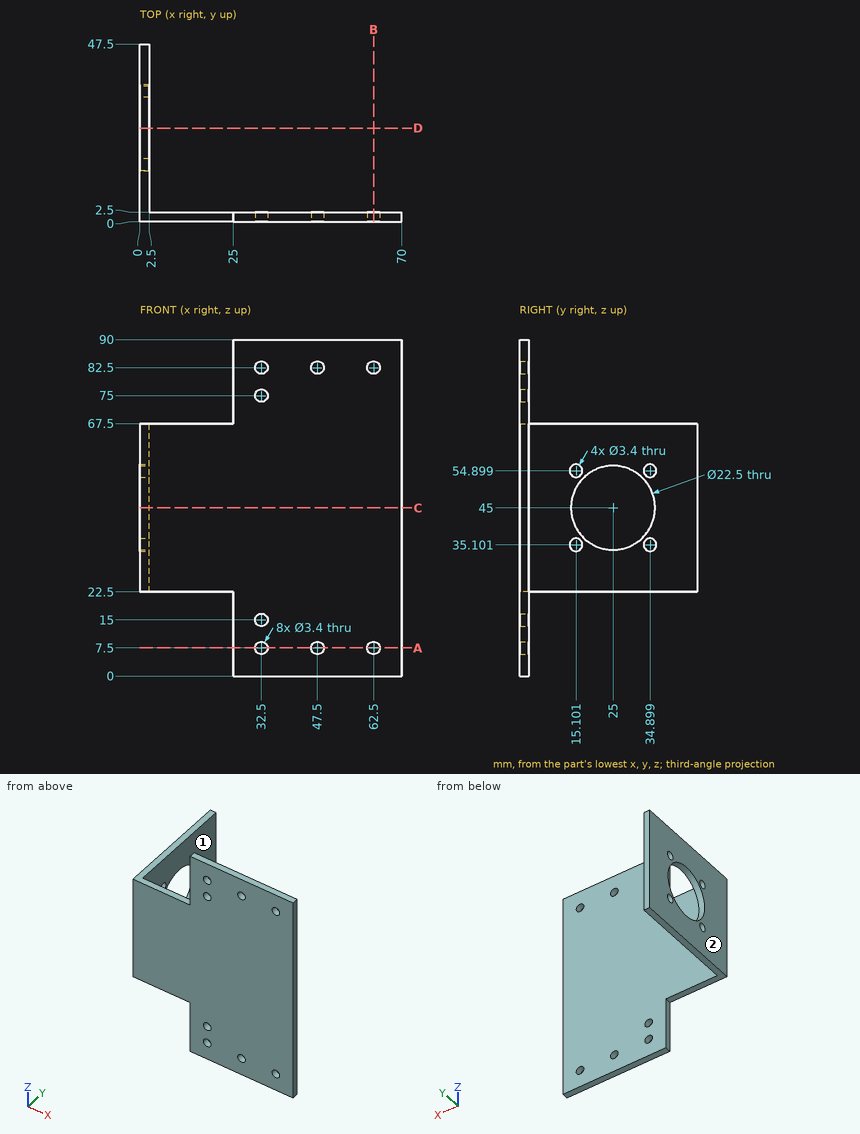
Check sheet for the drawn part. Datum: minimum x, y, z corner. Units: mm. A direction names the side the tool comes from. Coordinates: 2 decimals unless noted, no trailing zeros. Loops run counter-clockwise (first coordinate to the right, second up) from the corner with the lowest first, then second, coordinate; pieces in that order, holes last. Notation, with made-up numbers: (56, -0.5) -> (99, -0.5) arc R4 ccw to (99, 3.5) -> close; hole circle Ø8 at (59, -33). An arc over 180 degrees is marked (long way). Answer as a JSON object with one key per item and string values. Group by question number.
Item 1: Depth check by flat-ended pin: pin 1 (2 mm diameter, centred on y = 0.5, z = 78.5, fed in from -X); pin 2 (10 mm diameter, centred on x = 23.5, z = 67.5, fed in from +Y); pin 3 (2 mm diameter, centred on x = 47.5, z = 82.5, fed in from +Y); pin 4 (4 mm diameter, centred on y = 34, z = 56.5, fed in from +X). Enter the tip coordinate at first touch or a pass-through.
Item 2: Sectioned sample at B-B on x = 62.5. Record the boundary of the cut face in (y, z).
Item 3: Sectioned sample at A-A on z = 7.5. Record the boundary of the cut face in (x, y).
Item 4: Tool access check on the marked faces 1 and 2. Record the directions out of +Z, -Z, +X, -X, +Y, -Y that give a thin tool (end or side, any length) a straight path to the whole face; none if there is none.
Item 5: Scan lines: probe 1 along Z at (x, y) = (47.5, 1.4); probe 2 along X at (y, z) = (1, 82.5); probe 3 along Y at (x, z) = (40, 56.5). Record each from-to range of solid material in increasing order.
Item 6: Sectioned sample at C-C on z = 45. Record the boundary of the cut face in (x, y).
Item 7: Sectioned sample at D-D on y = 25. Record the boundary of the cut face in (x, z).
Evaluation:
{
 "1": {"pin 1": "stops at x = 25", "pin 2": "stops at y = 2.5", "pin 3": "passes through", "pin 4": "stops at x = 2.5"},
 "2": {"outline": "(0, 0) -> (2.5, 0) -> (2.5, 5.8) -> (0, 5.8) -> close; (0, 9.2) -> (2.5, 9.2) -> (2.5, 80.8) -> (0, 80.8) -> close; (0, 84.2) -> (2.5, 84.2) -> (2.5, 90) -> (0, 90) -> close"},
 "3": {"outline": "(25, 0) -> (30.8, 0) -> (30.8, 2.5) -> (25, 2.5) -> close; (34.2, 0) -> (45.8, 0) -> (45.8, 2.5) -> (34.2, 2.5) -> close; (49.2, 0) -> (60.8, 0) -> (60.8, 2.5) -> (49.2, 2.5) -> close; (64.2, 0) -> (70, 0) -> (70, 2.5) -> (64.2, 2.5) -> close"},
 "4": {"face 1": "+Z, -Z, +X, +Y", "face 2": "+Z, -Z, -X, +Y, -Y"},
 "5": {"probe 1": "z = 0 to 5.8, 9.2 to 80.8, 84.2 to 90", "probe 2": "x = 25 to 30.8, 34.2 to 45.8, 49.2 to 60.8, 64.2 to 70", "probe 3": "y = 0 to 2.5"},
 "6": {"outline": "(0, 0) -> (70, 0) -> (70, 2.5) -> (2.5, 2.5) -> (2.5, 13.75) -> (0, 13.75) -> close; (0, 36.25) -> (2.5, 36.25) -> (2.5, 47.5) -> (0, 47.5) -> close"},
 "7": {"outline": "(0, 22.5) -> (2.5, 22.5) -> (2.5, 33.75) -> (0, 33.75) -> close; (0, 56.25) -> (2.5, 56.25) -> (2.5, 67.5) -> (0, 67.5) -> close"}
}
